Print and shaded views of the part. All mm, measured from the part's lowest x, y and z. A direction names the side the tool comes from. Give positions to 0.01 mm unless a question says otherwise; leave off trailing zeros. Loops run counter-clockwise (first coordinate to the right, second up) from the corner with the lowest first, then second, coordinate; pieces in that order, holes last. Notation, with made-up numbers: (-22, 17) - (5, 17) arc R16 cw to (5, 24) - close; hole circle Ø3 at (-30, 18). An arc over 180 degrees is marked (long way). Return JSON: item names as keys, results as strings.
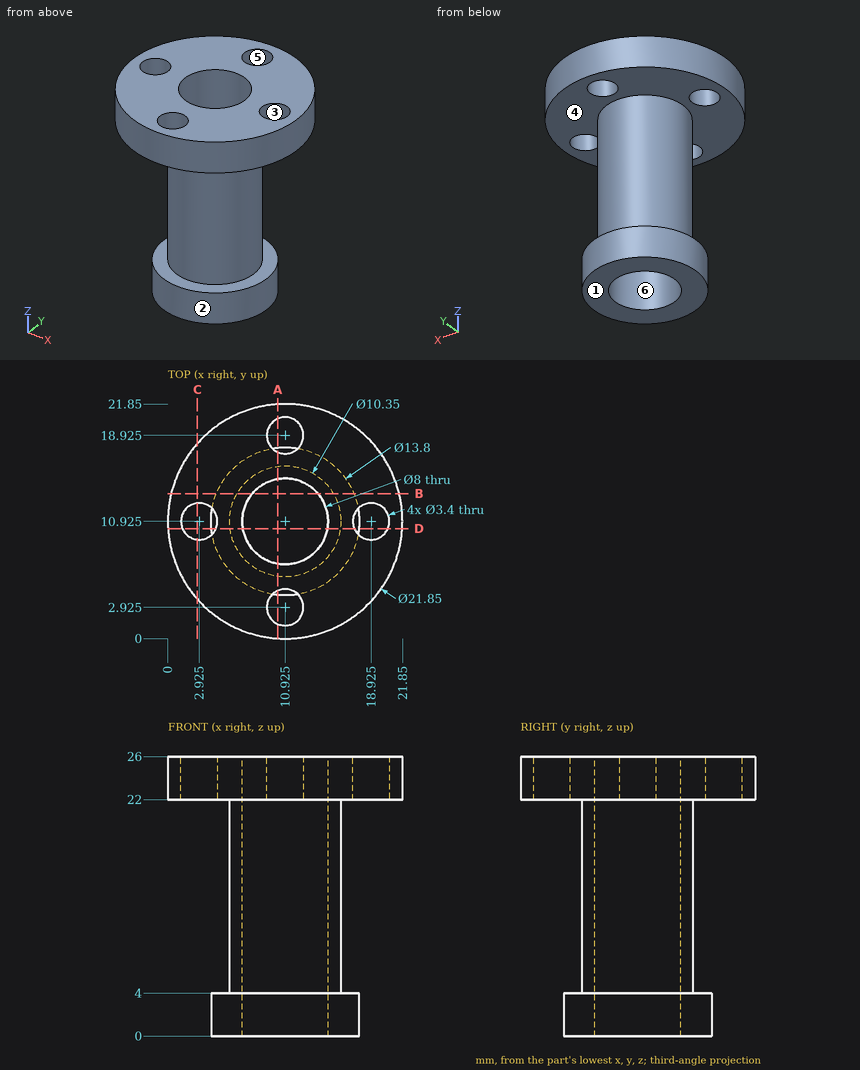
1. Drop flat-ended pins along their axis: P1, Ø1, axis at y = 16, z = 15.5, coming from the +X side; P2, Ø4, axis at x = 14, y = 11.5, coming from the +Z side; P3, Ø3, axis at y = 6.5, z = 4, coming from the +X side; P4, Ø5, axis at x = 15, z = 8.5, coming from the -Y side. Give the stop position or say it passes through.
Values follow:
{"P1": "stops at x = 13.34", "P2": "stops at z = 26", "P3": "stops at x = 17.17", "P4": "stops at y = 6"}
2. Which spindle directions (+Z, -Z, +X, -X, +Y, -Y) get a long thin tool onto all of the face, cutting with end or side? Do the marked faces 4, 5 and 6. Say none if no direction does.
Values follow:
{"face 4": "none", "face 5": "+Z", "face 6": "+Z, -Z"}
3. Drill centre lines: probe 1 along X at (y, z) = (11, 11); probe 2 along Z at (x, y) = (12, 17); probe 3 along X at (y, z) = (7.5, 5). Where is each one in solid material? Low to high.
Values follow:
{"probe 1": "x = 5.75 to 6.93, 14.92 to 16.1", "probe 2": "z = 0 to 4, 22 to 26", "probe 3": "x = 7.05 to 8.86, 12.99 to 14.8"}
4. Cut at C-C, the plane x = 2.75. Write the cut outline in (y, z).
Values follow:
{"outline": "(3.68, 22) - (9.23, 22) - (9.23, 26) - (3.68, 26) - close; (12.62, 22) - (18.17, 22) - (18.17, 26) - (12.62, 26) - close"}
5. Pull direction Y, two halves, no side cores. Call the marked faces 1, 2 and 3: +Y half, -Y half, draft (parallel to the pull), parting line (faces both ways), or undercut.
Values follow:
{"face 1": "draft", "face 2": "parting line", "face 3": "undercut"}
6. Cut at B-B, the plane y = 13.5. Write the cut outline in (x, z).
Values follow:
{"outline": "(0.31, 22) - (6.44, 22) - (6.44, 4) - (4.52, 4) - (4.52, 0) - (7.86, 0) - (7.86, 26) - (0.31, 26) - close; (13.99, 0) - (17.33, 0) - (17.33, 4) - (15.41, 4) - (15.41, 22) - (21.54, 22) - (21.54, 26) - (13.99, 26) - close"}
7. Cut at A-A, the plane x = 10.25. Write the cut outline in (y, z), plus the area to 3 significant figures.
Values follow:
{"outline": "(0.02, 22) - (1.36, 22) - (1.36, 26) - (0.02, 26) - close; (4.06, 0) - (6.98, 0) - (6.98, 26) - (4.49, 26) - (4.49, 22) - (5.79, 22) - (5.79, 4) - (4.06, 4) - close; (14.87, 0) - (17.79, 0) - (17.79, 4) - (16.06, 4) - (16.06, 22) - (17.36, 22) - (17.36, 26) - (14.87, 26) - close; (20.49, 22) - (21.83, 22) - (21.83, 26) - (20.49, 26) - close", "area": "96.9 mm²"}
